```python
from build123d import *

# Parameters (mm, degrees)
BOSS_EXTRUDE1_DEPTH = 10
BOSS_EXTRUDE2_DEPTH = 50
SKETCH3_R           = 13.5
BOSS_EXTRUDE3_DEPTH = 8
CHAMFER2_SIZE       = 5
FILLET1_R           = 25
CUT_EXTRUDE1_DEPTH  = 10


with BuildPart() as part:
    # Sketch1 → Boss-Extrude1 (new body)
    with BuildSketch(Plane(origin=(0, 0, 0), x_dir=(1, 0, 0), z_dir=(0, 1, 0))):
        with BuildLine():
            Line((30.30044843, 30.235426009), (1.30044843, 30.235426009))
            Line((1.30044843, 30.235426009), (1.30044843, 10.235426009))
            ThreePointArc((1.30044843, 10.235426009), (8.371516242, 7.306493821), (11.30044843, 0.235426009))
            ThreePointArc((11.30044843, 0.235426009), (8.371516242, -6.835641803), (1.30044843, -9.764573991))
            Line((1.30044843, -9.764573991), (1.30044843, -129.764573991))
            ThreePointArc((1.30044843, -129.764573991), (8.371516242, -132.693506179), (11.30044843, -139.764573991))
            ThreePointArc((11.30044843, -139.764573991), (8.371516242, -146.835641803), (1.30044843, -149.764573991))
            Line((1.30044843, -149.764573991), (1.30044843, -169.764573991))
            Line((1.30044843, -169.764573991), (30.30044843, -169.764573991))
            Line((30.30044843, -169.764573991), (30.30044843, 30.235426009))
        make_face()
        with BuildLine():
            Line((1.30044843, 10.235426009), (1.30044843, 30.235426009))
            Line((1.30044843, 30.235426009), (-27.69955157, 30.235426009))
            Line((-27.69955157, 30.235426009), (-27.69955157, -169.764573991))
            Line((-27.69955157, -169.764573991), (1.30044843, -169.764573991))
            Line((1.30044843, -169.764573991), (1.30044843, -149.764573991))
            ThreePointArc((1.30044843, -149.764573991), (-8.69955157, -139.764573991), (1.30044843, -129.764573991))
            Line((1.30044843, -129.764573991), (1.30044843, -9.764573991))
            ThreePointArc((1.30044843, -9.764573991), (-8.69955157, 0.235426009), (1.30044843, 10.235426009))
        make_face()
        with BuildLine():
            ThreePointArc((11.30044843, 0.235426009), (8.371516242, 7.306493821), (1.30044843, 10.235426009))
            Line((1.30044843, 10.235426009), (1.30044843, -9.764573991))
            ThreePointArc((1.30044843, -9.764573991), (8.371516242, -6.835641803), (11.30044843, 0.235426009))
        make_face()
        with BuildLine():
            Line((1.30044843, -9.764573991), (1.30044843, 10.235426009))
            ThreePointArc((1.30044843, 10.235426009), (-8.69955157, 0.235426009), (1.30044843, -9.764573991))
        make_face()
        with BuildLine():
            ThreePointArc((11.30044843, -139.764573991), (8.371516242, -132.693506179), (1.30044843, -129.764573991))
            Line((1.30044843, -129.764573991), (1.30044843, -149.764573991))
            ThreePointArc((1.30044843, -149.764573991), (8.371516242, -146.835641803), (11.30044843, -139.764573991))
        make_face()
        with BuildLine():
            Line((1.30044843, -149.764573991), (1.30044843, -129.764573991))
            ThreePointArc((1.30044843, -129.764573991), (-8.69955157, -139.764573991), (1.30044843, -149.764573991))
        make_face()
    extrude(amount=BOSS_EXTRUDE1_DEPTH)

    # Sketch1<3> → Boss-Extrude2 (add)
    with BuildSketch(Plane(origin=(0, 0, 0), x_dir=(1, 0, 0), z_dir=(0, 1, 0))):
        with BuildLine():
            ThreePointArc((11.30044843, 0.235426009), (8.371516242, 7.306493821), (1.30044843, 10.235426009))
            Line((1.30044843, 10.235426009), (1.30044843, -9.764573991))
            ThreePointArc((1.30044843, -9.764573991), (8.371516242, -6.835641803), (11.30044843, 0.235426009))
        make_face()
        with BuildLine():
            Line((1.30044843, -9.764573991), (1.30044843, 10.235426009))
            ThreePointArc((1.30044843, 10.235426009), (-8.69955157, 0.235426009), (1.30044843, -9.764573991))
        make_face()
        with BuildLine():
            ThreePointArc((11.30044843, -139.764573991), (8.371516242, -132.693506179), (1.30044843, -129.764573991))
            Line((1.30044843, -129.764573991), (1.30044843, -149.764573991))
            ThreePointArc((1.30044843, -149.764573991), (8.371516242, -146.835641803), (11.30044843, -139.764573991))
        make_face()
        with BuildLine():
            Line((1.30044843, -149.764573991), (1.30044843, -129.764573991))
            ThreePointArc((1.30044843, -129.764573991), (-8.69955157, -139.764573991), (1.30044843, -149.764573991))
        make_face()
    extrude(amount=BOSS_EXTRUDE2_DEPTH)

    # Sketch3 → Boss-Extrude3 (add)
    with BuildSketch(Plane(origin=(0, 50, 0), x_dir=(1, 0, 0), z_dir=(0, 1, 0))):
        with Locations(Location((1.30044843, -139.764573991, 0), (0, 0, 270))):
            Circle(SKETCH3_R)
        with Locations(Location((1.30044843, 0.235426009, 0), (0, 0, 270))):
            Circle(SKETCH3_R)
    extrude(amount=BOSS_EXTRUDE3_DEPTH)

    # Chamfer2
    # the kernel refuses this chamfer: 5 mm, written as the material it adds along each edge
    with BuildSketch(Plane(origin=(1.30044843, 50, -0.235426009), x_dir=(0, 0, -1), z_dir=(-1, 0, 0))) as chamfer2_piece_1_section:
        Polygon((10, CHAMFER2_SIZE), (10 + CHAMFER2_SIZE, 0), (10, 0), align=None)
    chamfer2_piece_1 = revolve(axis=Axis((1.30044843, 50, -0.235426009), (0, -1, 0)), mode=Mode.PRIVATE)
    chamfer2_piece_1 = chamfer2_piece_1 & Plane(origin=(1.30044843, 46.747090697, -0.235426009), x_dir=(0, 0, 1), z_dir=(0, -1, 0)) * Cylinder(13.5, 61, mode=Mode.PRIVATE)
    add(chamfer2_piece_1)
    with BuildSketch(Plane(origin=(1.30044843, 50, 139.764573991), x_dir=(0, 0, -1), z_dir=(-1, 0, 0))) as chamfer2_piece_2_section:
        Polygon((10 + CHAMFER2_SIZE, 0), (10, CHAMFER2_SIZE), (10, 0), align=None)
    chamfer2_piece_2 = revolve(axis=Axis((1.30044843, 50, 139.764573991), (0, -1, 0)), mode=Mode.PRIVATE)
    chamfer2_piece_2 = chamfer2_piece_2 & Plane(origin=(1.30044843, 46.747090697, 139.764573991), x_dir=(0, 0, 1), z_dir=(0, -1, 0)) * Cylinder(13.5, 60, mode=Mode.PRIVATE)
    add(chamfer2_piece_2)

    # Fillet1
    fillet1_edges = [part.edges().sort_by_distance(p)[0] for p in [
        (-27.69955157, 5, -30.235426009),
        (30.30044843, 5, -30.235426009),
        (30.30044843, 5, 169.764573991),
        (-27.69955157, 5, 169.764573991),
    ]]
    fillet(fillet1_edges, radius=FILLET1_R)

    # Sketch4 → Cut-Extrude1 (cut)
    with BuildSketch(Plane(origin=(0, 10, 0), x_dir=(1, 0, 0), z_dir=(0, 1, 0))):
        with BuildLine():
            ThreePointArc((4.30044843, 21.985426009), (3.421768774, 24.106746353), (1.30044843, 24.985426009))
            Line((1.30044843, 24.985426009), (1.30044843, 18.985426009))
            ThreePointArc((1.30044843, 18.985426009), (3.421768774, 19.864105665), (4.30044843, 21.985426009))
        make_face()
        with BuildLine():
            Line((1.30044843, 18.985426009), (1.30044843, 24.985426009))
            ThreePointArc((1.30044843, 24.985426009), (-1.69955157, 21.985426009), (1.30044843, 18.985426009))
        make_face()
        with BuildLine():
            ThreePointArc((4.30044843, -69.764573991), (3.421768774, -67.643253647), (1.30044843, -66.764573991))
            Line((1.30044843, -66.764573991), (1.30044843, -72.764573991))
            ThreePointArc((1.30044843, -72.764573991), (3.421768774, -71.885894335), (4.30044843, -69.764573991))
        make_face()
        with BuildLine():
            Line((1.30044843, -72.764573991), (1.30044843, -66.764573991))
            ThreePointArc((1.30044843, -66.764573991), (-1.69955157, -69.764573991), (1.30044843, -72.764573991))
        make_face()
        with BuildLine():
            ThreePointArc((4.30044843, -161.514573991), (3.421768774, -159.393253647), (1.30044843, -158.514573991))
            Line((1.30044843, -158.514573991), (1.30044843, -164.514573991))
            ThreePointArc((1.30044843, -164.514573991), (3.421768774, -163.635894335), (4.30044843, -161.514573991))
        make_face()
        with BuildLine():
            Line((1.30044843, -164.514573991), (1.30044843, -158.514573991))
            ThreePointArc((1.30044843, -158.514573991), (-1.69955157, -161.514573991), (1.30044843, -164.514573991))
        make_face()
    extrude(amount=-CUT_EXTRUDE1_DEPTH, mode=Mode.SUBTRACT)


solid = part.part
```
Part model, mm, in its own coordinate system. A direction names the side the tool comes from. Round coordinates to 2 decimals unless told otherwise and drop trailing zeros. Order: outer loops, then holes, each group sorted by start corner. A loop starts at its lowest first (then second) coordinate and runs counter-clockwise, first axis right, second up. Notation, with made-up numbers: M 23.25,-19 L 57.25,-19 A19 ccw 57.25,-6 Z; hole C 53.5,12 d5. An arc over 180 degrees is marked long. Put each result on its own line as item: value. Start each with the question number.
1. Tool access for faces 5 (the face through (-7.77, 45.22, -4.95)), 6 (the face through (1, 5, -30.235)), 7 (the face through (-2.755, 53.183, 152.641)): list every direction of +Z, -Z, +X, -X, +Y, -Y with a clear straight run to the whole face (end or side of a thin tool).
2. Slice it at A-A on y = 7. List the corners of the cut face in (x, z).
3. Slice it at D-D on x = -22. List the corners of the cut face in (y, z), then the cut area to 3 significant figures.
4. Two-plate mould, pull along Z, no slides. Class faces 1 (the face through (7, 10, 68)), 2 (the face through (-20.57, 5.07, -22.72)), 3 (the face through (-4.888, 45.17, 147.835)), 4 (the face through (-20.18, 5.07, 162.64)): +Z half, -Z half, draft (parallel to the pull), parting line (faces both ways), or undercut.
5. Drop flat-ended pins along their axis: pin 1 (8 mm diameter, centred on x = -12, y = 8.5, fed in from -Z); pin 2 (1.5 mm diameter, centred on x = -8, y = 39, fed in from +Z); pin 3 (1 mm diameter, centred on x = -8.5, z = 31, fed in from +Y). Give the stop position or say it passes through.
6. Drill centre lines: probe 1 along Y at (x, z) = (16.5, 98.5); probe 2 along Z at (x, y) = (-6.5, 48.5); probe 3 along Z at (x, y) = (-7.5, 12). Where is each one in solid material? Low to high. Write a range as [from, to].
7. Slice it at C-C on z = 108.5. List the corners of the cut face in (x, y).
8. Slice it at B-B on y = 35. List the corners of the cut face in (x, z), then the cut area to 3 significant figures.
Findings:
1. face 5: none
1. face 6: -Z, +X, -X, +Y, -Y
1. face 7: +Y
2. outline: M -27.7,-5.24 A25 ccw -2.7,-30.24 L 5.3,-30.24 A25 ccw 30.3,-5.24 L 30.3,144.76 A25 ccw 5.3,169.76 L -2.7,169.76 A25 ccw -27.7,144.76 Z; hole C 1.3,-21.99 d6; hole C 1.3,69.76 d6; hole C 1.3,161.51 d6
3. outline: M 0,-21.13 L 10,-21.13 L 10,160.65 L 0,160.65 Z
3. area: 1,820 mm2
4. face 1: undercut
4. face 2: -Z half
4. face 3: undercut
4. face 4: +Z half
5. pin 1: z = -29.67
5. pin 2: z = 144.95
5. pin 3: y = 10
6. probe 1: [0, 10]
6. probe 2: [-11.25, 10.78], [128.75, 150.78]
6. probe 3: [-4.98, 4.51], [135.02, 144.51]
7. outline: M -27.7,0 L 30.3,0 L 30.3,10 L -27.7,10 Z
8. outline: C 1.3,-0.24 d20; C 1.3,139.76 d20
8. area: 628 mm2
